```python
from build123d import *

# Parameters (mm, degrees)
SKETCH1_R           = 4
SKETCH1_R_2         = 1.5
BOSS_EXTRUDE2_DEPTH = 5


with BuildPart() as part:
    # Sketch1 → Boss-Extrude2 (new body)
    with BuildSketch(Plane.XY):
        with BuildLine():
            Line((220, -10), (220, -12))
            ThreePointArc((220, -12), (220.878679656, -14.121320344), (223, -15))
            Line((223, -15), (240, -15))
            ThreePointArc((240, -15), (247.071067812, -12.071067812), (250, -5))
            Line((250, -5), (250, 5))
            ThreePointArc((250, 5), (247.071067812, 12.071067812), (240, 15))
            Line((240, 15), (223, 15))
            ThreePointArc((223, 15), (220.878679656, 14.121320344), (220, 12))
            Line((220, 12), (220, 10))
            Line((220, 10), (18.874586088, 10))
            ThreePointArc((18.874586088, 10), (15.181841359, 10.706796227), (12.011100238, 12.727272727))
            ThreePointArc((12.011100238, 12.727272727), (-17.5, 0), (12.011100238, -12.727272727))
            ThreePointArc((12.011100238, -12.727272727), (15.181841359, -10.706796227), (18.874586088, -10))
            Line((18.874586088, -10), (220, -10))
        make_face()
        Circle(SKETCH1_R, mode=Mode.SUBTRACT)
        with Locations((9.5, 0)):
            Circle(SKETCH1_R_2, mode=Mode.SUBTRACT)
        with Locations((-9.5, 0)):
            Circle(SKETCH1_R_2, mode=Mode.SUBTRACT)
        with Locations((0, 8)):
            Circle(SKETCH1_R_2, mode=Mode.SUBTRACT)
        with Locations((0, -8)):
            Circle(SKETCH1_R_2, mode=Mode.SUBTRACT)
        with Locations((227.928932188, 7.071067812)):
            Circle(SKETCH1_R_2, mode=Mode.SUBTRACT)
        with Locations(Location((242.071067812, -7.071067812, 0), (0, 0, 180))):
            Circle(SKETCH1_R_2, mode=Mode.SUBTRACT)
        with Locations((242.071067812, 7.071067812)):
            Circle(SKETCH1_R_2, mode=Mode.SUBTRACT)
        with Locations(Location((227.928932188, -7.071067812, 0), (0, 0, 180))):
            Circle(SKETCH1_R_2, mode=Mode.SUBTRACT)
    extrude(amount=BOSS_EXTRUDE2_DEPTH)


solid = part.part
```
Input: part model. Units: mm. Frame: model coordinates. A direction names the side the tool comes from. Give positions to 0.01 mm unless a question says otherwise; leave off trailing zeros. Order: outer loops, then holes, each group sorted by start corner. A loop starts at its lowest first (then second) coordinate and runs counter-clockwise, first axis right, second up. Notation, with made-up numbers: (8, 6.25) -> (55, 6.25) arc R22 ccw to (55, 12.25) -> close; hole circle Ø3 at (61, 41.25). An arc over 180 degrees is marked (long way). Write each question's results on one line, items separated by ' | '. Start each with the question number.
Item 1: Cut plane B-B on x = 195. Return the cut outline in (y, z).
Item 2: Set-up query: faces 4 (the flat face through (232, 15, 2)), 5 (the flat face through (114, 0, 5)), 6 (the cylindrical face through (15.2, 10.7, 2.5)), 7 (the flat face through (118, -10, 2)), 8 (the flat face through (231, -15, 2)). Return all of +Z, -Z, +X, -X, +Y, -Y with unobstructed straight access to the full face (end or side cutting, diameter ignored); none if empty.
Item 3: Line query: line 1 (Y direction, x = 0, z = 3.5); line 2 (X direction, y = -0.5, z = 2.75); line 3 (Y direction, x = 188, z = 3.85). Output: solid intervals per line, ascending.
Item 4: Cut plane A-A on z = 3.5. Give the number of separate pieces and of enclosed holes in the cut face, then the cut area to 3 significant figures.
Item 5: Contact query for flat-ended pins moving along their axis: P1, Ø1.5, axis at x = 157.5, z = 3, coming from the +Y side; P2, Ø1.5, axis at x = 231, z = 1.5, coming from the -Y side; P3, Ø9, axis at x = 0, y = 0, coming from the -Z side; P4, Ø2.5, axis at x = 158.5, z = 1.5, coming from the -Y side. Output: stop coordinate, or through.
Item 6: Mould query, pull axis Y, two halves, no side actions, for faces 1 (the cylindrical face through (-0.867, -3.905, 2.465)), 2 (the cylindrical face through (247.15, 11.99, 2.46)), 3 (the flat face through (250, 0, 2)). Classes: pulls with the +Y half, pulls with the -Y half, needs draft (parallel to the pull), parting line crosses it, or undercut.
Established:
1) outline: (-10, 0) -> (10, 0) -> (10, 5) -> (-10, 5) -> close
2) face 4: +Z, -Z, +X, +Y | face 5: +Z, +X, -X, +Y, -Y | face 6: +Z, -Z, +Y | face 7: +Z, -Z, -Y | face 8: +Z, -Z, +X, -Y
3) line 1: -17.5 to -9.5, -6.5 to -4, 4 to 6.5, 9.5 to 17.5 | line 2: -17.49 to -10.91, -8.09 to -3.97, 3.97 to 8.09, 10.91 to 250 | line 3: -10 to 10
4) separate pieces: 1 | enclosed holes: 9 | area: 5,780 mm^2
5) P1: y = 10 | P2: y = -15 | P3: z = 0 | P4: y = -10
6) face 1: undercut | face 2: pulls with the +Y half | face 3: needs draft
